Check sheet for the modelled part. Datum: model origin and axes. Units: mm. A direction names the side the tool comes from. Round coordinates to 2 decimals unless told otherwise and drop trailing zeros. Order: outer loops, then holes, each group sorted by start corner. A loop starts at its lowest first (then second) coordinate and runs counter-clockwise, first axis right, second up. Notation, with made-up numbers: (27.25, -33) -> (48.25, -33) arc R26 ccw to (48.25, -16) -> close; hole circle Ø1 at (49.5, 47). An arc over 180 degrees is marked (long way). Answer in a Markdown table with one row per item. Add a question column.
1. Access from +Z, -Z, +X, -X, +Y, -Y to the whole of each face (thin tool, end or side, straight path). Record for faces 1 (the flat face through (-6, -3, 0)), 2 (the flat face through (10, -0.176, 10)), 3 (the cylindrical face through (9.605, 8.323, 17.01)), 4 (the cylindrical face through (4.42, 7.43, 0.27)).
2. Sectioned sample at A-A, the plane x = -9.5. Record the boundary of the cut face in (y, z).
3. Sectioned sample at D-D, the plane x = 1.5. Record the boundary of the cut face in (y, z), then the cut area to 3 significant figures.
4. Sectioned sample at B-B, the plane y = 2. Record the boundary of the cut face in (x, z).
5. Draft check along X on faces 5 (the cylindrical face through (-0.04, 7.46, -1.48)), 6 (the cylindrical face through (-3.805, 13.727, -1.479)), 7 (the flat face through (11, 7, 22)). Enter one of: +X half, -X half, draft (parallel to the pull), parting line (faces both ways), or undercut.
6. Material ranges on L1, parallel to X at y = 10, z = -0.5; L2, parallel to Z at x = -4, y = -5; L3, parallel to Y at x = 6.5, z = -0.5, recorded low to high. Write a range as from..to.
7. Sectioned sample at C-C, the plane z = 10.5. Record the boundary of the cut face in (x, y), then the cut area to 3 significant figures.
8. Depth check by flat-ended pin: P1, Ø15.5, axis at x = -9.5, y = -5.5, coming from the +Z side; P2, Ø1, axis at x = 0, y = -9.5, coming from the +Z side; P3, Ø12, axis at y = -2, z = 18, coming from the -X side; P4, Ø3.5, axis at x = 9, z = 8.5, coming from the -Y side. Enter the tip coordinate at first touch or a pass-through.
```python
from build123d import *

# Parameters (mm, degrees)
F0_R     = 1.4
F0_W     = 10
F0_H     = 15
F3_DEPTH = 3
F2_W     = 8
F2_H     = 15
F5_R     = 2
F5_R_2   = 1
F6_DEPTH = 10
F7_DEPTH = 15
F8_R     = 1


with BuildPart() as f3:
    # F0 (on Top) → F3 (new body)
    with BuildSketch(Plane.XY):
        with BuildLine():
            Line((-2.3220218662, -1.1490219488), (4.1030128133, -18.2824477607))
            ThreePointArc((4.1030128133, -18.2824477607), (11.8277285282, -21.7936821766), (15.3389629441, -14.0689664616))
            Line((15.3389629441, -14.0689664616), (5.9639629441, 10.9310335384))
            ThreePointArc((5.9639629441, 10.9310335384), (3.7635569052, 13.7558465942), (0.3459878787, 14.8242928889))
            Line((0.3459878787, 14.8242928889), (-4.6540121213, 14.8242928889))
            Line((-4.6540121213, 14.8242928889), (-4.6540121213, -0.1757071111))
            Line((-4.6540121213, -0.1757071111), (-3.7265156326, -0.1757071111))
            ThreePointArc((-3.7265156326, -0.1757071111), (-2.8721233759, -0.4428186848), (-2.3220218662, -1.1490219488))
        make_face()
        with Locations((9.7209878787, -16.1757071111)):
            Circle(F0_R, mode=Mode.SUBTRACT)
        with Locations((0.3459878787, 8.8242928889)):
            Circle(F0_R, mode=Mode.SUBTRACT)
        with Locations((-9.6540121213, 7.3242928889)):
            Rectangle(F0_W, F0_H)
    extrude(amount=-F3_DEPTH)

    # F0 (on Top) → F4 section 0
    with BuildSketch(Plane.XY):
        with Locations((-9.6540121213, 7.3242928889)):
            Rectangle(F0_W, F0_H)
    # F2 (on offset) → F4 section 1
    with BuildSketch(Plane.XY.offset(22)):
        with Locations((-10.5001659675, 7.3242928889)):
            Rectangle(F2_W, F2_H)
    loft()

    # F5 (on face) → F6 (join)
    with BuildSketch(Plane(origin=(-14.6532955437, 0, 0.1024705982), x_dir=(0, -1, 0), z_dir=(-0.9999755498, 0, 0.006992836))):
        with Locations((-7.3242928889, 16.8980648133)):
            Circle(F5_R)
        with Locations((-7.3242928889, 16.8980648133)):
            Circle(F5_R_2, mode=Mode.SUBTRACT)
    extrude(amount=-F6_DEPTH)

    # F5 (on face) → F7 (cut)
    with BuildSketch(Plane(origin=(-14.6532955437, 0, 0.1024705982), x_dir=(0, -1, 0), z_dir=(-0.9999755498, 0, 0.006992836))):
        with Locations((-7.3242928889, 16.8980648133)):
            Circle(F5_R_2)
    extrude(amount=-F7_DEPTH, mode=Mode.SUBTRACT)

    # F8
    f8_edges = [f3.edges().sort_by_distance(p)[0] for p in [
        (-6.500166, 7.324293, 22),
        (-14.500166, 7.324293, 22),
        (-4.654012, 7.324293, 0),
    ]]
    fillet(f8_edges, radius=F8_R)


with BuildPart() as f9_1:
    # F9: instance of F3
    add(f3.part.mirror(Plane.YZ))


solid = f9_1.part
```
Answer key:
| question | item | result |
|---|---|---|
| 1 | face 1 | +Z, -X, +Y, -Y |
| 1 | face 2 | +Z, -Z, +X, -Y |
| 1 | face 3 | none |
| 1 | face 4 | -X, +Y, -Y |
| 2 | outline | (-22.17, -3) -> (-17.56, -3) -> (-17.56, 0) -> (-22.17, 0) -> close; (-14.79, -3) -> (1.5, -3) -> (1.5, 0) -> (-14.79, 0) -> close |
| 3 | outline | (-3.34, -3) -> (14.82, -3) -> (14.82, 0) -> (-3.34, 0) -> close |
| 3 | area | 54.5 mm² |
| 4 | outline | (-9.31, -3) -> (14.65, -3) -> (14.65, 0) -> (14.51, 21.01) arc R1 ccw to (13.51, 22) -> (7.42, 22) arc R1 ccw to (6.42, 21.08) -> (4.73, 0.92) arc R1 cw to (3.73, 0) -> (-9.31, 0) -> close |
| 5 | face 5 | undercut |
| 5 | face 6 | -X half |
| 5 | face 7 | draft |
| 6 | L1 | x = -6.31..-1.11, 0.41..14.65 |
| 6 | L2 | z = -3..0 |
| 6 | L3 | y = -0.18..14.82 |
| 7 | outline | (5.54, -0.18) -> (14.58, -0.18) -> (14.58, 14.82) -> (5.54, 14.82) -> close |
| 7 | area | 136 mm² |
| 8 | P1 | stops at z = 0 |
| 8 | P2 | passes through |
| 8 | P3 | stops at x = 5.68 |
| 8 | P4 | stops at y = -0.18 |
